Design review of the part built by this model. Coordinates are the model's own, in mm. Face numbers are marked on the shaded views. A direction names the side the tool comes from. Coordinates: 2 decimals unless noted, no trailing zeros. Write each loop counter-clockwise with the first axis right and the second up, starting at its lowest first coordinate (ties: lowest second). Pieces come first, ordered by that corner, then holes.
Q1. Machinability: for the marked faces 1, 2 and 3, which of the approach directions +Z, -Z, +X, -X, +Y, -Y give a long, thin tool a straight path to every point of the face, cutting with its end or side? Answer none if there is none.
Q2. The part is to be moulded in two halves that separate along Y. For the marked faces 4, 5, 6 and 7, say which applies: +Y half, -Y half, draft (parallel to the pull), parting line (faces both ways), or undercut.
Q3. Add section C-C, the plane z = 26. Give the number of separate pieces and of enclosed holes in the cut face, plus the area to 3 significant figures.
Q4. Add section A-A, the plane y = 15. Give the boundary of the cut face in (x, z), plus the area to 3 significant figures.
Q5. To check wall thickness, follow probe 1 along Y at (x, z) = (23.5, 30.5); probe 2 along X at (y, z) = (-55, 18); probe 3 along Y at (x, z) = (-27.5, 17.5). State the ranges of each line that lie inside material, in increasing order.
Q6. Add section B-B, the plane y = -64. Give the boundary of the cut face in (x, z), plus the area to 3 significant figures.
Q7. Clearance check with flat-ended pins moving along their axes: pin 1 Ø12 at (x, y) = (-34.5, -29) entering from -Z; pin 2 Ø18 at (x, z) = (-34.5, 18) entering from -Y; pin 3 Ø3 at (x, y) = (42, 27) entering from +Z; pin 4 Ø10.5 at (x, z) = (-51.5, 18) entering from -Y. State where each tip first meets the part, or that it passes through.
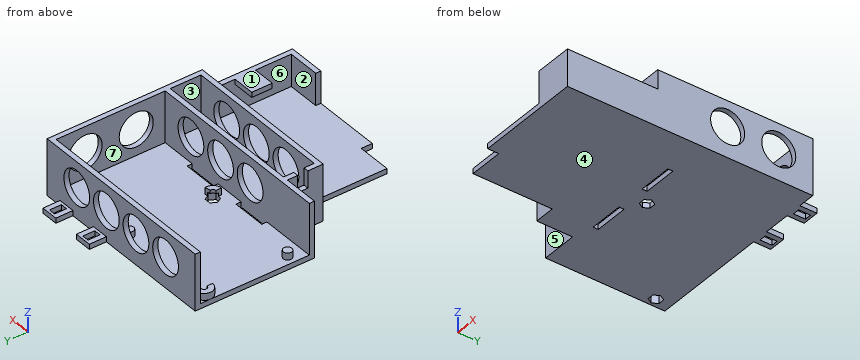
Solid Edge part; units mm, degrees
sketch "Sketch1" plane through (0, 0, 0) normal (0, 0, 1) x (1, 0, 0)
  line L0 (57.5, -35) -> (-57.5, -35)
  line L1 (-57.5, -35) -> (-57.5, 35)
  line L2 (-57.5, 35) -> (57.5, 35)
  line L3 (57.5, 35) -> (57.5, -35)
extrude "Protrusion1" add sketch "Sketch1" along normal blind 3
sketch "Sketch2" plane through (0, 0, 3) normal (0, 0, 1) x (1, 0, 0)
  circle A0 centre (-52.5, -23) radius 2.5
  circle A1 centre (5.5, 26) radius 2.5
  circle A2 centre (5.5, -23) radius 5
  circle A3 centre (5.5, -23) radius 1.75
  circle A4 centre (-52.5, 26) radius 1.75
  circle A5 centre (-52.5, 26) radius 5
extrude "ExtrudedProtrusion_2" add sketch "Sketch2" along normal blind 4
sketch "Sketch3" plane through (0, 0, 3) normal (0, 0, 1) x (1, 0, 0)
  line L0 (-52.5, 26) -> (-52.5, 21)
  line L1 (-52.5, 26) -> (-48.9645, 29.5355)
  arc A0 (-48.9645, 29.5355) -> (-52.5, 21) centre (-52.5, 26) cw
  line L2 (5.5, -23) -> (5.5, -28)
  line L3 (5.5, -23) -> (10.4282, -22.1558)
  arc A1 (5.5, -28) -> (10.4282, -22.1558) centre (5.5, -23) cw
extrude "ExtrudedCutout_1" cut sketch "Sketch3" along normal blind 4
sketch "Sketch4" plane through (0, 0, 3) normal (0, 0, 1) x (1, 0, 0)
  line L0 (-48.8338, 26) -> (-50.6669, 29.175)
  line L1 (-50.6669, 29.175) -> (-54.3331, 29.175)
  line L2 (-54.3331, 29.175) -> (-56.1662, 26)
  line L3 (-56.1662, 26) -> (-54.3331, 22.825)
  line L4 (-54.3331, 22.825) -> (-50.6669, 22.825)
  line L5 (-50.6669, 22.825) -> (-48.8338, 26)
  line L6 (1.8338, -23) -> (3.6669, -26.175)
  line L7 (3.6669, -26.175) -> (7.3331, -26.175)
  line L8 (7.3331, -26.175) -> (9.1662, -23)
  line L9 (9.1662, -23) -> (7.3331, -19.825)
  line L10 (7.3331, -19.825) -> (3.6669, -19.825)
  line L11 (3.6669, -19.825) -> (1.8338, -23)
extrude "Cutout1" cut sketch "Sketch4" against normal up to vertex (3 mm away)
sketch "Sketch5" plane through (0, 0, 3) normal (0, 0, 1) x (1, 0, 0)
  line L0 (-50.6669, 22.825) -> (-48.8338, 26)
  line L1 (-48.8338, 26) -> (-50.6669, 29.175)
  line L2 (-50.6669, 29.175) -> (-54.3331, 29.175)
  line L3 (-54.3331, 29.175) -> (-56.1662, 26)
  line L4 (-56.1662, 26) -> (-54.3331, 22.825)
  line L5 (-54.3331, 22.825) -> (-50.6669, 22.825)
extrude "ExtrudedCutout_3" cut sketch "Sketch5" along normal blind 2
sketch "Sketch6" plane through (0, 0, 3) normal (0, 0, 1) x (1, 0, 0)
  line L0 (1.8338, -23) -> (3.6669, -26.175)
  line L1 (3.6669, -26.175) -> (7.3331, -26.175)
  line L2 (7.3331, -26.175) -> (9.1662, -23)
  line L3 (9.1662, -23) -> (7.3331, -19.825)
  line L4 (7.3331, -19.825) -> (3.6669, -19.825)
  line L5 (3.6669, -19.825) -> (1.8338, -23)
extrude "ExtrudedCutout_4" cut sketch "Sketch6" along normal blind 2
extrude "ExtrudedCutout_5" [suppressed]
sketch "Sketch7" plane through (0, 0, 3) normal (0, 0, 1) x (1, 0, 0)
  line L0 (57.5, -35) -> (-57.5, -35)
  line L1 (-57.5, -35) -> (-57.5, -32)
  line L2 (-57.5, -32) -> (54.5, -32)
  line L3 (54.5, 32) -> (54.5, -32)
  line L4 (-57.5, 32) -> (54.5, 32)
  line L5 (-57.5, 35) -> (-57.5, 32)
  line L6 (57.5, 35) -> (-57.5, 35)
  line L7 (57.5, 32) -> (57.5, 35)
  line L8 (57.5, 32) -> (57.5, -35)
extrude "ExtrudedProtrusion_6" add sketch "Sketch7" along normal blind 30
sketch "Sketch8" plane through (0, 0, 0) normal (0, 0, -1) x (1, 0, 0)
  line L0 (37.5, -45) -> (47.5, -45)
  line L1 (47.5, -45) -> (47.5, -35)
  line L2 (47.5, -35) -> (37.5, -35)
  line L3 (37.5, -35) -> (37.5, -45)
  line L4 (40.5, -43.5) -> (44.5, -43.5)
  line L5 (44.5, -43.5) -> (44.5, -36.5)
  line L6 (44.5, -36.5) -> (40.5, -36.5)
  line L7 (40.5, -36.5) -> (40.5, -43.5)
  line L8 (11.5, -45) -> (21.5, -45)
  line L9 (21.5, -45) -> (21.5, -35)
  line L10 (21.5, -35) -> (11.5, -35)
  line L11 (11.5, -35) -> (11.5, -45)
  line L12 (14.5, -43.5) -> (18.5, -43.5)
  line L13 (18.5, -43.5) -> (18.5, -36.5)
  line L14 (18.5, -36.5) -> (14.5, -36.5)
  line L15 (14.5, -36.5) -> (14.5, -43.5)
extrude "ExtrudedProtrusion_7" add sketch "Sketch8" against normal blind 3
sketch "Sketch9" plane through (-0.75, -35, 16.5) normal (0, -1, 0) x (1, 0, 0)
  circle A0 centre (-33.75, 1.5) radius 10
  circle A1 centre (-10.75, 1.5) radius 10
  circle A2 centre (12.25, 1.5) radius 10
  circle A3 centre (35.25, 1.5) radius 10
extrude "Cutout2" cut sketch "Sketch9" against normal up to vertex (70 mm away)
sketch "Sketch10" plane through (57.5, 0.75, 16.5) normal (1, 0, 0) x (0, 1, 0)
  circle A0 centre (-15.75, 1.5) radius 10
  circle A1 centre (14.25, 1.5) radius 10
extrude "Cutout3" cut sketch "Sketch10" against normal up to vertex (3 mm away)
sketch "Sketch11" plane through (0, 5, 0) normal (0, 0, -1) x (1, 0, 0)
  line L0 (-36.5, 40) -> (-36.5, 61)
  line L1 (57.5, 61) -> (-36.5, 61)
  line L2 (57.5, 40) -> (57.5, 61)
  line L3 (57.5, 40) -> (-36.5, 40)
extrude "ExtrudedProtrusion_10" add sketch "Sketch11" against normal blind 3
sketch "Sketch12" plane through (10.5, -45.5, 3) normal (0, 0, 1) x (1, 0, 0)
  line L0 (-44, -7.5) -> (44, -7.5)
  line L1 (44, -7.5) -> (44, 10.5)
  line L2 (44, 10.5) -> (47, 10.5)
  line L3 (47, 10.5) -> (47, -10.5)
  line L4 (47, -10.5) -> (-47, -10.5)
  line L5 (-47, -10.5) -> (-47, 10.5)
  line L6 (-47, 10.5) -> (-44, 10.5)
  line L7 (-44, 10.5) -> (-44, -7.5)
extrude "Protrusion2" add sketch "Sketch12" along normal up to vertex (30 mm away)
sketch "Sketch13" plane through (-0.75, -35, 16.5) normal (0, -1, 0) x (1, 0, 0)
  circle A0 centre (-33.75, 1.5) radius 10
extrude "Protrusion3" add sketch "Sketch13" against normal up to vertex (3 mm away)
sketch "Sketch14" plane through (-0.75, -35, 16.5) normal (0, -1, 0) x (1, 0, 0)
  circle A0 centre (35.25, 1.5) radius 10
  circle A1 centre (12.25, 1.5) radius 10
  circle A2 centre (-10.75, 1.5) radius 10
extrude "Cutout4" cut sketch "Sketch14" along normal up to vertex (21 mm away)
sketch "Sketch15" plane through (0, 0, 0) normal (0, 0, 1) x (1, 0, 0)
  line L0 (-24.5, -109) -> (57.5, -109)
  line L1 (57.5, -109) -> (57.5, -56)
  line L2 (57.5, -56) -> (-24.5, -56)
  line L3 (-24.5, -56) -> (-24.5, -109)
extrude "Protrusion4" add sketch "Sketch15" along normal up to vertex (3 mm away)
sketch "Sketch16" plane through (13.5, -82, 3) normal (0, 0, 1) x (0, -1, 0)
  line L0 (24, 22) -> (24, 41)
  line L1 (24, 41) -> (-26, 41)
  line L2 (-26, 41) -> (-26, 44)
  line L3 (-26, 44) -> (27, 44)
  line L4 (27, 44) -> (27, 22)
  line L5 (27, 22) -> (24, 22)
extrude "ExtrudedProtrusion_18" add sketch "Sketch16" along normal blind 18.75
extrude "ExtrudedProtrusion_13" [suppressed]
sketch "Sketch17" plane through (-36.5, -45.5, 16.5) normal (-1, 0, 0) x (0, -1, 0)
  line L0 (-1.5, 6.5) -> (1.5, 6.5)
  line L1 (1.5, 6.5) -> (1.5, 16.5)
  line L2 (1.5, 16.5) -> (-1.5, 16.5)
  line L3 (-4.5, 16.5) -> (-1.5, 16.5)
  line L4 (-4.5, 6.5) -> (-4.5, 16.5)
  line L5 (-1.5, 6.5) -> (-4.5, 6.5)
extrude "ExtrudedCutout_12" cut sketch "Sketch17" against normal blind 3
sketch "Sketch18" plane through (-1.5, 0, 3) normal (0, 0, 1) x (0, -1, 0)
  line L0 (29, 15) -> (32, 15)
  line L1 (32, 15) -> (32, 35)
  line L2 (32, 35) -> (29, 35)
  line L3 (29, 35) -> (29, 15)
  line L4 (32, -3) -> (29, -3)
  line L5 (29, -3) -> (29, -23)
  line L6 (29, -23) -> (32, -23)
  line L7 (32, -23) -> (32, -3)
  line L8 (109, -3) -> (102.5, -3)
  line L9 (102.5, -3) -> (102.5, -23)
  line L10 (102.5, -23) -> (109, -23)
  line L11 (109, -23) -> (109, -3)
extrude "ExtrudedCutout_13" cut sketch "Sketch18" against normal blind 3
sketch "Sketch19" plane through (54.5, -84.5, 13) normal (-1, 0, 0) x (0, -1, 0)
  line L0 (0.5, 5.75) -> (-11.5, 5.75)
  line L1 (-11.5, 5.75) -> (-11.5, 8.75)
  line L2 (-11.5, 8.75) -> (0.5, 8.75)
  line L3 (0.5, 8.75) -> (0.5, 5.75)
extrude "ExtrudedProtrusion_19" add sketch "Sketch19" along normal blind 13
fillet "Round_2" [suppressed]
fillet "Round_3" [suppressed]
extrude "Cutout5" [suppressed]
extrude "Cutout6" [suppressed]
fillet "Round_4" [suppressed]
fillet "Round_5" [suppressed]
Here are the results:
1. face 1: +Z, +X, -X, -Y
1. face 2: +Z, -X
1. face 3: +Z
2. face 4: draft
2. face 5: -Y half
2. face 6: undercut
2. face 7: undercut
3. separate pieces: 13
3. enclosed holes: 0
3. area: 822 mm2
4. outline: (-57.5, 0) - (57.5, 0) - (57.5, 8) - (54.5, 8) - (54.5, 3) - (-57.5, 3) - close; (54.5, 28) - (57.5, 28) - (57.5, 33) - (54.5, 33) - close
4. area: 375 mm2
5. probe 1: y = -56 to -53, -35 to -32, 32 to 35
5. probe 2: x = -36.5 to -21.5, -1.5 to 1.5, 21.5 to 24.5, 44.5 to 57.5
5. probe 3: y = -56 to -53, -35 to -32
6. outline: (-24.5, 0) - (57.5, 0) - (57.5, 21.75) - (54.5, 21.75) - (54.5, 3) - (-24.5, 3) - close
6. area: 302 mm2
7. pin 1: stops at z = 0
7. pin 2: stops at y = -56
7. pin 3: stops at z = 3
7. pin 4: stops at y = -35
